For this review, take the finished solid that the model builds, in its own axes (mm). A direction names the side the tool comes from. Give positions to 0.01 mm unless a question says otherwise; leave off trailing zeros. Write each loop counter-clockwise with the first axis right and the second up, starting at its lowest first coordinate (ties: lowest second). Pieces come first, ordered by that corner, then holes. Notation, with made-up numbers: M 18,32 L 66,32 A11 cw 66,48 Z; hole C 6,35 d9. An arc over 180 degrees is marked long. One line per item, written item: value. Start each with the question number.
Item 1: Consider section B-B, the plane y = -19. Write out the cut boundary in (x, z).
Item 2: Clearance check with flat-ended pins moving along their axes: pin 1 Ø4 at (x, z) = (-47.5, 15.5) entering from -Y; pin 2 Ø3 at (y, z) = (86, 8.5) entering from +X; pin 3 Ø12 at (x, z) = (-0.5, 5.5) entering from +Y (3 decimals). State where each tip first meets the part, or that it passes through.
Item 3: Mouldability with a two-part tool opening along Y and no side actions: class faces 3 (the face through (23, 115, 30)), 4 (the face through (-64.907, 27.581, 9.86)), 5 (the face through (14.387, -23.644, 9.86)), 6 (the face through (27.264, -3.593, 23.819)) as released by +Y, released by -Y, zero draft, split by the parting line, or undercut.
Item 4: To check wall thickness, follow probe 1 along Y at (x, z) = (0, 8.5); probe 2 along Y at (x, z) = (17, 6.75); probe 3 along X at (y, z) = (1, 16). State the ranges of each line that lie inside material, in increasing order.
Item 5: Tool access review of faces 1 (the face through (-0.78, -13.05, 15.21)), 2 (the face through (-47.6, 119.83, 18.12)): name each direction out of +Z, -Z, +X, -X, +Y, -Y from which nothing blocks a thin tool from reaching the whole face with its end or side.
Item 6: Consider section C-C, the plane x = -19. Write out the cut boundary in (y, z).
Item 7: Consider section A-A, the plane z = 25. Give the number of separate pieces and of enclosed holes in the cut face, and give its area (3 significant figures).
Item 8: Consider section D-D, the plane x = 20.5. Write out the cut boundary in (y, z), and give its area (3 significant figures).
```python
from build123d import *

# Parameters (mm, degrees)
SKETCH1_R               = 27.5
SKETCH1_R_2             = 19
SKETCH1_R_3             = 10
BOSS_EXTRUDE1_DEPTH     = 30
SKETCH2_R               = 20
SKETCH2_R_2             = 15
BOSS_EXTRUDE2_DEPTH     = 30
BOSS_EXTRUDE2_2_DEPTH   = 30
SKETCH5_R               = 6
CUT_EXTRUDE1_DEPTH      = 30
BOSS_EXTRUDE3_DEPTH     = 20
SKETCH7_R               = 15
SKETCH7_R_2             = 6
SKETCH7_R_3             = 10
CUT_EXTRUDE2_DEPTH      = 11
CUT_EXTRUDE2_DEPTH_BACK = 21


with BuildPart() as part:
    # Sketch1 → Boss-Extrude1 (new body)
    with BuildSketch(Plane.XY):
        Circle(SKETCH1_R)
        Circle(SKETCH1_R_2, mode=Mode.SUBTRACT)
        Circle(SKETCH1_R_2)
        Circle(SKETCH1_R_3, mode=Mode.SUBTRACT)
    extrude(amount=BOSS_EXTRUDE1_DEPTH)

    # Sketch5 → Cut-Extrude1 (cut)
    with BuildSketch(Plane.XY):
        with Locations((0, 19)):
            Circle(SKETCH5_R)
        with Locations((-19, 0)):
            Circle(SKETCH5_R)
        with Locations((0, -19)):
            Circle(SKETCH5_R)
        with Locations((19, 0)):
            Circle(SKETCH5_R)
    extrude(amount=CUT_EXTRUDE1_DEPTH, mode=Mode.SUBTRACT)



with BuildPart() as body_2:
    # Sketch2 → Boss-Extrude2 (new body)
    with BuildSketch(Plane.XY):
        with Locations((-45, 100)):
            Circle(SKETCH2_R)
        with Locations((-45, 100)):
            Circle(SKETCH2_R_2, mode=Mode.SUBTRACT)
    extrude(amount=BOSS_EXTRUDE2_DEPTH)


with BuildPart() as body_3:
    # Sketch2 → Boss-Extrude2 2 (new body)
    with BuildSketch(Plane.XY):
        with Locations((20, 100)):
            Circle(SKETCH2_R)
        with Locations((20, 100)):
            Circle(SKETCH2_R_2, mode=Mode.SUBTRACT)
    extrude(amount=BOSS_EXTRUDE2_2_DEPTH)


with BuildPart() as part_1:
    add(part.part)

    add(body_2.part)  # Boss-Extrude3 merges body 2

    add(body_3.part)  # Boss-Extrude3 merges body 3
    # Sketch6 → Boss-Extrude3 (add)
    with BuildSketch(Plane.XY):
        with BuildLine():
            Line((35.914568173, 87.886927728), (27.176428779, -4.206152493))
            ThreePointArc((27.176428779, -4.206152493), (14.094792579, -23.82005481), (-9.394166008, -25.845689099))
            ThreePointArc((-9.394166008, -25.845689099), (-66.335656198, 31.148009393), (-61.323361203, 111.556291751))
            ThreePointArc((-61.323361203, 111.556291751), (-45, 119.870223993), (-28.676638797, 111.556291751))
            ThreePointArc((-28.676638797, 111.556291751), (-12.5, 103.317089225), (3.676638797, 111.556291751))
            ThreePointArc((3.676638797, 111.556291751), (31.685854827, 115.916260455), (35.914568173, 87.886927728))
        make_face()
    extrude(amount=BOSS_EXTRUDE3_DEPTH)

    # Sketch7 → Cut-Extrude2 (cut, two sides)
    with BuildSketch(Plane.XY.offset(20)) as cut_extrude2_sk:
        with Locations((-45, 100)):
            Circle(SKETCH7_R)
        with Locations((20, 100)):
            Circle(SKETCH7_R)
        with Locations((0, 19)):
            Circle(SKETCH7_R_2)
        with Locations((-19, 0)):
            Circle(SKETCH7_R_2)
        with Locations((0, -19)):
            Circle(SKETCH7_R_2)
        with Locations((19, 0)):
            Circle(SKETCH7_R_2)
        Circle(SKETCH7_R_3)
    extrude(amount=CUT_EXTRUDE2_DEPTH, mode=Mode.SUBTRACT)
    extrude(cut_extrude2_sk.sketch, amount=-CUT_EXTRUDE2_DEPTH_BACK, mode=Mode.SUBTRACT)


solid = part_1.part
```
Model answer:
1. outline: M -23.8,0 L -6,0 L -6,30 L -19.88,30 L -19.88,20 L -23.8,20 Z; M 6,0 L 20.1,0 L 20.1,20 L 19.88,20 L 19.88,30 L 6,30 Z
2. pin 1: stops at y = -1.93
2. pin 2: stops at x = 35.88
2. pin 3: stops at y = 113.775
3. face 3: zero draft
3. face 4: split by the parting line
3. face 5: released by -Y
3. face 6: undercut
4. probe 1: y = -27.61 to -25, -13 to -10, 10 to 13, 25 to 107.7
4. probe 2: y = -21.84 to -5.66, 5.66 to 85.3, 114.7 to 119.77
4. probe 3: x = -48.19 to -24.92, -13.08 to -9.95, 9.95 to 13.08, 24.92 to 27.67
5. face 1: +Z, -Z
5. face 2: +Z
6. outline: M -21.6,0 L -6,0 L -6,30 L -19.88,30 L -19.88,20 L -21.6,20 Z; M 6,0 L 104.4,0 L 104.4,20 L 19.88,20 L 19.88,30 L 6,30 Z
7. separate pieces: 3
7. enclosed holes: 7
7. area: 2,710 mm2
8. outline: M -18.56,0 L -5.81,0 L -5.81,30 L -18.33,30 L -18.33,20 L -18.56,20 Z; M 5.81,0 L 85.01,0 L 85.01,30 L 80.01,30 L 80.01,20 L 18.33,20 L 18.33,30 L 5.81,30 Z; M 114.99,0 L 119.99,0 L 119.99,30 L 114.99,30 Z
8. area: 2,290 mm2
